```python
from build123d import *

# Parameters (mm, degrees)
SALIENTE_EXTRUIR1_DEPTH            = 50
CORTAR_EXTRUIR1_DEPTH              = 72
CORTAR_EXTRUIR4_REACH              = 144.211
CROQUIS6_W                         = 30
CROQUIS6_H                         = 25
CORTAR_EXTRUIR5_REACH              = 144.211
CROQUIS8_W                         = 30
CROQUIS8_H                         = 30
CORTAR_EXTRUIR6_DEPTH              = 40
CROQUIS9_W                         = 30
CROQUIS9_H                         = 30
CORTAR_EXTRUIR7_DEPTH              = 40
CROQUIS10_W                        = 6.35
CROQUIS10_H                        = 12.9
CORTAR_EXTRUIR8_DEPTH              = 33
CORTAR_EXTRUIR9_REACH              = 144.211
CORTAR_EXTRUIR10_REACH             = 144.211
CORTAR_EXTRUIR10_DIRECTION_2_DEPTH = 143.210791725
CROQUIS14_W                        = 12.6
CROQUIS14_H                        = 18
CORTAR_EXTRUIR11_DEPTH             = 5
CROQUIS15_W                        = 12.517773713
CROQUIS15_H                        = 18.001366708
CORTAR_EXTRUIR12_DEPTH             = 5
CROQUIS16_W                        = 7.6
CROQUIS16_H                        = 2.5
CORTAR_EXTRUIR13_DEPTH             = 9
CORTAR_EXTRUIR14_DEPTH             = 1.8


with BuildPart() as part:
    # Croquis1 → Saliente-Extruir1 (new body)
    with BuildSketch(Plane(origin=(0, 0, 0), x_dir=(1, 0, 0), z_dir=(0, 1, 0))):
        Polygon((-96.830741331, 0), (96.830741331, 0), (96.830741331, 63), (36, 91.365840534), (-36, 91.365840534), (-96.830741331, 63), align=None)
    extrude(amount=SALIENTE_EXTRUIR1_DEPTH)

    # Croquis3D2 → Cortar-Extruir1 (cut)
    with BuildSketch(Plane(origin=(-36, 0, -91.365840534), x_dir=(0, 0.6600783810393928, 0.751196732477195), z_dir=(-1, 0, 0))):
        Polygon((0, 0), (58.835678645, -11.762776814), (93.598994681, 0), (40.781406688, 46.410941988), align=None)
    extrude(amount=-CORTAR_EXTRUIR1_DEPTH, mode=Mode.SUBTRACT)

    # Cortar-Barrer1: sweep along a curve in space
    with BuildLine() as cortar_barrer1_path:
        Line((96.830741331, 50, -63), (36, 50, -91.365840534))
    # Croquis2 → Cortar-Barrer1 (sweep, cut)
    with BuildSketch(Plane.ZY.offset(-36)):
        Polygon((-91.365840534, 50), (-27.857310923, 50), (-39.404316307, 30), (-91.365840534, 0), align=None)
    sweep(path=cortar_barrer1_path.line, mode=Mode.SUBTRACT)

    # Cortar-Barrer2: sweep along a curve in space
    with BuildLine() as cortar_barrer2_path:
        Line((-36, 50, -91.365840534), (-96.830741331, 50, -63))
    # Croquis3 → Cortar-Barrer2 (sweep, cut)
    with BuildSketch(Plane(origin=(-36, 0, 0), x_dir=(0, 0, -1), z_dir=(1, 0, 0))):
        Polygon((27.857310923, 50), (91.365840534, 50), (91.365840534, 0), (39.404316307, 30), align=None)
    sweep(path=cortar_barrer2_path.line, mode=Mode.SUBTRACT)

    # Croquis6 → Cortar-Extruir4 (cut, up to next)
    with BuildSketch(Plane.XY, mode=Mode.PRIVATE) as cortar_extruir4_sk1:
        with Locations((0, 37.5)):
            Rectangle(CROQUIS6_W, CROQUIS6_H)
    cortar_extruir4_tool1 = extrude(cortar_extruir4_sk1.sketch, amount=-CORTAR_EXTRUIR4_REACH, mode=Mode.PRIVATE) & part.part
    add(cortar_extruir4_tool1.solids().sort_by_distance((0, 37.5, 0))[0], mode=Mode.SUBTRACT)

    # Croquis7 → Cortar-Extruir5 (cut, up to next)
    with BuildSketch(Plane(origin=(0, 50, 0), x_dir=(1, 0, 0), z_dir=(0, 1, 0)), mode=Mode.PRIVATE) as cortar_extruir5_sk1:
        Polygon((-36, 13.928655461), (36, 13.928655461), (65.87009803, 0), (-65.87009803, 0), align=None)
    cortar_extruir5_tool1 = extrude(cortar_extruir5_sk1.sketch, amount=-CORTAR_EXTRUIR5_REACH, mode=Mode.PRIVATE) & part.part
    add(cortar_extruir5_tool1.solids().sort_by_distance((0, 50, -6.28364))[0], mode=Mode.SUBTRACT)

    # Croquis8 → Cortar-Extruir6 (cut)
    with BuildSketch(Plane(origin=(-11.764807584, 0, -25.229711282), x_dir=(0.9063077870366527, 0, -0.4226182617406937), z_dir=(0.4226182617406937, 0, 0.9063077870366527))):
        with Locations((-46.740576174, 35)):
            Rectangle(CROQUIS8_W, CROQUIS8_H)
    extrude(amount=-CORTAR_EXTRUIR6_DEPTH, mode=Mode.SUBTRACT)

    # Croquis9 → Cortar-Extruir7 (cut)
    with BuildSketch(Plane(origin=(11.764807584, 0, -25.229711282), x_dir=(0.9063077870366495, 0, 0.42261826174070066), z_dir=(-0.42261826174070066, 0, 0.9063077870366495))):
        with Locations((46.740576174, 35)):
            Rectangle(CROQUIS9_W, CROQUIS9_H)
    extrude(amount=-CORTAR_EXTRUIR7_DEPTH, mode=Mode.SUBTRACT)

    # Croquis10 → Cortar-Extruir8 (cut)
    with BuildSketch(Plane.XY.offset(-13.928655461)):
        with Locations((-21.525, 11.451366708)):
            Rectangle(CROQUIS10_W, CROQUIS10_H)
        with Locations((21.525, 11.451366708)):
            Rectangle(CROQUIS10_W, CROQUIS10_H)
    extrude(amount=-CORTAR_EXTRUIR8_DEPTH, mode=Mode.SUBTRACT)

    # Croquis12 → Cortar-Extruir9 (cut, up to next)
    with BuildSketch(Plane(origin=(0, 50, 0), x_dir=(1, 0, 0), z_dir=(0, 1, 0)), mode=Mode.PRIVATE) as cortar_extruir9_sk1:
        Polygon((-96.830741331, 0), (-95.030741331, 0), (-95.030741331, 63.839353785), (-96.830741331, 63), align=None)
    cortar_extruir9_tool1 = extrude(cortar_extruir9_sk1.sketch, amount=-CORTAR_EXTRUIR9_REACH, mode=Mode.PRIVATE) & part.part
    add(cortar_extruir9_tool1.solids().sort_by_distance((-95.928756, 50, -31.710301))[0], mode=Mode.SUBTRACT)

    # Croquis13 → Cortar-Extruir10 (cut, up to next)
    with BuildSketch(Plane(origin=(0, 50, 0), x_dir=(1, 0, 0), z_dir=(0, 1, 0)), mode=Mode.PRIVATE) as cortar_extruir10_sk1:
        Polygon((96.830741331, 0), (95.032124755, 0), (95.032124755, 63.838708683), (96.830741331, 63), align=None)
    cortar_extruir10_tool1 = extrude(cortar_extruir10_sk1.sketch, amount=-CORTAR_EXTRUIR10_REACH, mode=Mode.PRIVATE) & part.part
    add(cortar_extruir10_tool1.solids().sort_by_distance((95.929451, 50, -31.710139))[0], mode=Mode.SUBTRACT)

    # Croquis13 → Cortar-Extruir10 direction 2 (cut)
    with BuildSketch(Plane(origin=(0, 50, 0), x_dir=(1, 0, 0), z_dir=(0, 1, 0))):
        Polygon((96.830741331, 0), (95.032124755, 0), (95.032124755, 63.838708683), (96.830741331, 63), align=None)
    extrude(amount=CORTAR_EXTRUIR10_DIRECTION_2_DEPTH, mode=Mode.SUBTRACT)

    # Croquis14 → Cortar-Extruir11 (cut)
    with BuildSketch(Plane(origin=(95.032124755, 0, 0), x_dir=(0, 0, -1), z_dir=(1, 0, 0))):
        with Locations((6.3, 9)):
            Rectangle(CROQUIS14_W, CROQUIS14_H)
    extrude(amount=-CORTAR_EXTRUIR11_DEPTH, mode=Mode.SUBTRACT)

    # Croquis15 → Cortar-Extruir12 (cut)
    with BuildSketch(Plane.ZY.offset(95.030741331)):
        with Locations((-6.258886857, 9.000683354)):
            Rectangle(CROQUIS15_W, CROQUIS15_H)
    extrude(amount=-CORTAR_EXTRUIR12_DEPTH, mode=Mode.SUBTRACT)

    # Croquis16 → Cortar-Extruir13 (cut)
    with BuildSketch(Plane.XZ):
        with Locations((-81.230741331, -1.25)):
            Rectangle(CROQUIS16_W, CROQUIS16_H)
        with Locations((81.232124755, -1.25)):
            Rectangle(CROQUIS16_W, CROQUIS16_H)
    extrude(amount=-CORTAR_EXTRUIR13_DEPTH, mode=Mode.SUBTRACT)

    # Croquis17 → Cortar-Extruir14 (cut)
    with BuildSketch(Plane.XZ):
        Polygon((-81.230741331, -2.5), (-84.730741331, -2.5), (-84.730741331, -13.5), (-77.730741331, -13.5), (-77.730741331, -2.5), align=None)
        Polygon((77.730741331, -13.5), (77.730741331, -2.5), (81.230741331, -2.5), (84.730741331, -2.5), (84.730741331, -13.5), align=None)
    extrude(amount=-CORTAR_EXTRUIR14_DEPTH, mode=Mode.SUBTRACT)


solid = part.part
```
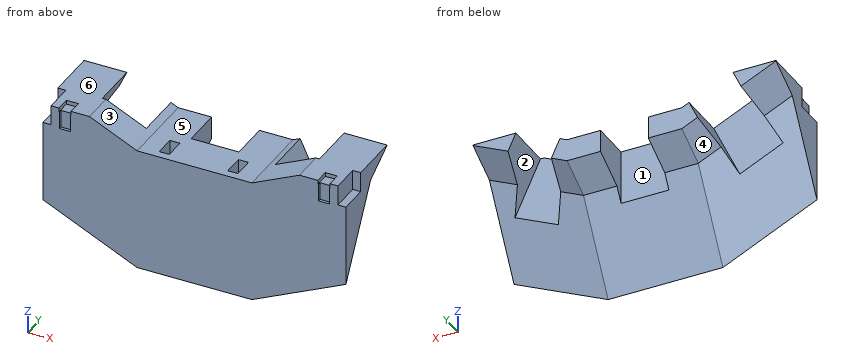
Here's how the part is built. I have some questions about the finished solid (model axes, mm). Face numbers are marked on the shaded views. A direction names the side the tool comes from. Coordinates: 2 decimals unless noted, no trailing zeros. Loops run counter-clockwise (first coordinate to the right, second up) from the corner with the lowest first, then second, coordinate; pieces in that order, holes last. Notation, with made-up numbers: (-6, 77.5) - (28, 77.5) arc R18 cw to (28, 90.5) - close; hole circle Ø1 at (31.5, 0.5). An arc over 180 degrees is marked (long way). Answer as CSV lines item,"result".
Q1. If we section it at B-B, the plane z = -6: Write out the boundary of the cut face in (x, y).
Response:
outline,"(-95.03, 18) - (-90.03, 18) - (-90.03, 0) - (-84.73, 0) - (-84.73, 1.8) - (-77.73, 1.8) - (-77.73, 0) - (-53, 0) - (-53, 20) - (-70.92, 20) - (-70.92, 50) - (-82.87, 50) - (-95.03, 40.18) - close; (53, 0) - (77.73, 0) - (77.73, 1.8) - (84.73, 1.8) - (84.73, 0) - (90.03, 0) - (90.03, 18) - (95.03, 18) - (95.03, 40.18) - (82.87, 50) - (70.92, 50) - (70.92, 20) - (53, 20) - close"
Q2. For the marked faces 1, 2 and 3, which set-ups out of +Z, -Z, +X, -X, +Y, -Y let a thin tool reach every point of the face, with its end or its side?
Response:
face 1,"+Z, -Z, +Y"
face 2,"-Z, +Y"
face 3,"+Z, +Y, -Y"
Q3. For pin 1 (1.5 mm diameter, centred on y = 45, z = -21.5, fed in from +X); pin 2 (8 mm diameter, centred on x = 16.5, y = 40, fed in from +Z); pin 3 (1.5 mm diameter, centred on x = 93.5, y = 12, fed in from +Z); pin 4 (14 mm diameter, centred on y = 4.5, z = -6.5, fed in from -X), each with a flat end and sliding along its axis, tell me the tip position at first contact or that it passes through.
Response:
pin 1,"x = 45.4"
pin 2,"z = -13.93"
pin 3,"z = -12.6"
pin 4,"x = -95.03"
Q4. If we section it at C-C, the plane x = -80.5: Write out the boundary of the cut face in (y, z).
Response:
outline,"(0, -70.62) - (20, -35.97) - (20, -26.54) - (25.45, -26.54) - (30, -18.65) - (50, -7.11) - (50, 0) - (9, 0) - (9, -2.5) - (1.8, -2.5) - (1.8, -13.5) - (0, -13.5) - close"
Q5. We'd pull the mould along X, two halves only. Please class the marked faces 4, 5 and 6: pulls with the +X half, pulls with the -X half, needs draft (parallel to the pull), parting line crosses it, or undercut.
Response:
face 4,"pulls with the -X half"
face 5,"undercut"
face 6,"needs draft"
Q6. If we section it at D-D, the plane y = 12: Write out the boundary of the cut face in (x, z).
Response:
outline,"(-95.03, -43.05) - (-36, -70.58) - (36, -70.58) - (95.03, -43.05) - (95.03, -12.6) - (90.03, -12.6) - (90.03, 0) - (65.87, 0) - (36, -13.93) - (24.7, -13.93) - (24.7, -46.93) - (18.35, -46.93) - (18.35, -13.93) - (-18.35, -13.93) - (-18.35, -46.93) - (-24.7, -46.93) - (-24.7, -13.93) - (-36, -13.93) - (-65.87, 0) - (-90.03, 0) - (-90.03, -12.52) - (-95.03, -12.52) - close"
Q7. If I drill on L1, parallel to X at y = 23, z = -19; L2, parallel to Y at x = 2.5, z = -33.5; L3, parallel to X at y = 22.5, z = -24.5, over which ranges is the centre line in solid material (lowest first)? Write a range as [from, to].
Response:
L1,"[-95.03, -76.98], [-43.88, 43.88], [76.98, 95.03]"
L2,"[0, 25]"
L3,"[-95.03, -79.55], [-46.45, 46.45], [79.55, 95.03]"
Q8. If we section it at A-A, the plane y = 27: Write out the boundary of the cut face in (x, z).
Response:
outline,"(-95.03, -17.07) - (-79.47, -24.33) - (-68.12, 0) - (-95.03, 0) - close; (-52.28, -37.01) - (-36, -44.6) - (-15, -44.6) - (-15, -13.93) - (-36, -13.93) - (-40.53, -11.82) - close; (15, -44.6) - (36, -44.6) - (52.28, -37.01) - (40.53, -11.82) - (36, -13.93) - (15, -13.93) - close; (68.12, 0) - (79.47, -24.33) - (95.03, -17.07) - (95.03, 0) - close"
